Read the model definition and answer for the solid it produces. Units are mm, in the model's axes. A direction names the side the tool comes from. Coordinates: 2 decimals unless noted, no trailing zeros. Loops run counter-clockwise (first coordinate to the right, second up) from the corner with the lowest first, then second, coordinate; pieces in that order, holes last. Notation, with made-up numbers: M 72.25,13 L 110.25,13 A25 ccw 110.25,41 Z; hole C -23,54 d7. An arc over 180 degrees is marked long. One line per item, written item: value. Start each with the question number.
1. The part is cut by section D-D (x = -114.5). Write down the section's boundary in (y, z), then the cut area to 3 significant figures.
2. The part is cut by section B-B (x = -17). Write down the section's boundary in (y, z).
3. For faces 4 (the face through (-144, 110, -7)), 5 (the face through (-144, -110, -7)), 6 (the face through (131.93, -37.13, -4.93)), 7 (the face through (-161, -100, 0)), 8 (the face through (-144, -90, -7)), determine the directions among +Z, -Z, +X, -X, +Y, -Y from which every point of the face is accessible in a straight line to the end or side of a thin tool.
4. Determine the mould class of faces 1 (the face through (-2, -20, 0)), 2 (the face through (-177.26, 99.86, -14.67)), 3 (the face through (-146.445, -190.979, 7.395)) for opening direction X: +X half, -X half, draft (parallel to the pull), parting line (faces both ways), or undercut.
5. Flat-ended cylindrical pins translate along their axes: pin 1 (4 mm diameter, centred on x = 122.5, z = -12, fed in from -Y); pin 2 (4 mm diameter, centred on y = 21, z = -12.5, fed in from +X); pin 3 (10 mm diameter, centred on x = -158.5, y = -97, fed in from +Z); pin 4 (5 mm diameter, centred on y = 48, z = 2, fed in from -X). Find the tip coordinate at first contact, or state that the pin passes through.
6. The part is cut by section C-C (y = -66). Write down the section's boundary in (x, z), then the cut area to 3 significant figures.
7. Consider probe 1 along Z at (x, y) = (-167, -103); probe 2 along X at (y, z) = (-98, -12.5); probe 3 along Z at (x, y) = (-106, -58). Determine where each line is inside the solid, lowest interval first.
8. The part is cut by section A-A (y = 24). Write down the section's boundary in (x, z).
```python
from build123d import *

# Parameters (mm, degrees)
BOSS_EXTRUDE1_DEPTH      = 15
BOSS_EXTRUDE2_DEPTH      = 10
BOSS_EXTRUDE2_DEPTH_BACK = 10
SKETCH3_R                = 12.5
SKETCH3_R_2              = 10
BOSS_EXTRUDE3_DEPTH      = 10
BOSS_EXTRUDE3_DEPTH_BACK = 10
SKETCH4_R                = 12.5
SKETCH4_R_2              = 10
CUT_EXTRUDE1_DEPTH       = 46
SKETCH6_R                = 7.5
BOSS_EXTRUDE4_DEPTH      = 10
BOSS_EXTRUDE5_DEPTH      = 5


with BuildPart() as part:
    # Sketch1 → Boss-Extrude1 (new body)
    with BuildSketch(Plane.XY):
        Polygon((-155, 155), (-155, -200), (155, -200), (155, 81.722524266), (81.722524266, 155), align=None)
    extrude(amount=BOSS_EXTRUDE1_DEPTH)

    # Sketch3 → Boss-Extrude2 (add, two sides: drawn at the far end of the back side and taken through both)
    # profile 1 of 2: a face of its own
    with BuildSketch(Plane(origin=(0, 100, 0), x_dir=(1, 0, 0), z_dir=(0, 1, 0)).offset(-BOSS_EXTRUDE2_DEPTH_BACK)):
        with BuildLine():
            ThreePointArc((-155, 12.5), (-158.661165235, 3.661165235), (-167.5, 0))
            Line((-167.5, 0), (-107.5, 0))
            Line((-107.5, 0), (-162.508319468, 23.960066556))
            ThreePointArc((-162.508319468, 23.960066556), (-157.04423588, 19.350328216), (-155, 12.5))
        make_face()
    # profile 2 of 2: a face of its own
    with BuildSketch(Plane(origin=(0, 100, 0), x_dir=(1, 0, 0), z_dir=(0, 1, 0)).offset(-BOSS_EXTRUDE2_DEPTH_BACK)):
        with Locations((-167.5, 12.5)):
            Circle(SKETCH3_R)
        with Locations(Location((-167.5, 12.5, 0), (0, 0, 270))):
            Circle(SKETCH3_R_2, mode=Mode.SUBTRACT)
    extrude(amount=BOSS_EXTRUDE2_DEPTH + BOSS_EXTRUDE2_DEPTH_BACK)

    # Sketch4 → Boss-Extrude3 (add, two sides: drawn at the far end of the back side and taken through both)
    # profile 1 of 2: a face of its own
    with BuildSketch(Plane(origin=(0, -100, 0), x_dir=(1, 0, 0), z_dir=(0, 1, 0)).offset(-BOSS_EXTRUDE3_DEPTH_BACK)):
        with Locations((-167.5, 12.5)):
            Circle(SKETCH4_R)
        with Locations(Location((-167.5, 12.5, 0), (0, 0, 270))):
            Circle(SKETCH4_R_2, mode=Mode.SUBTRACT)
    # profile 2 of 2: a face of its own
    with BuildSketch(Plane(origin=(0, -100, 0), x_dir=(1, 0, 0), z_dir=(0, 1, 0)).offset(-BOSS_EXTRUDE3_DEPTH_BACK)):
        with BuildLine():
            Line((-107.5, 0), (-162.508319468, 23.960066556))
            ThreePointArc((-162.508319468, 23.960066556), (-157.04423588, 19.350328216), (-155, 12.5))
            ThreePointArc((-155, 12.5), (-158.661165235, 3.661165235), (-167.5, 0))
            Line((-167.5, 0), (-107.5, 0))
        make_face()
    extrude(amount=BOSS_EXTRUDE3_DEPTH + BOSS_EXTRUDE3_DEPTH_BACK)

    # Sketch5 → Cut-Extrude1 (cut)
    with BuildSketch(Plane(origin=(0, 0, 0), x_dir=(-1, 0, 0), z_dir=(0, 0, -1))):
        with BuildLine():
            ThreePointArc((-125, -200), (-146.213203436, -191.213203436), (-155, -170))
            Line((-155, -170), (-155, -200))
            Line((-155, -200), (-125, -200))
        make_face()
        with BuildLine():
            ThreePointArc((155, -170), (146.213203436, -191.213203436), (125, -200))
            Line((125, -200), (155, -200))
            Line((155, -200), (155, -170))
        make_face()
        with BuildLine():
            Line((155, 155), (125, 155))
            ThreePointArc((125, 155), (146.213203436, 146.213203436), (155, 125))
            Line((155, 125), (155, 155))
        make_face()
        with BuildLine():
            Line((-81.722524266, 155), (-90.50932083, 146.213203436))
            ThreePointArc((-90.50932083, 146.213203436), (-80.776620365, 152.716385975), (-69.296117394, 155))
            Line((-69.296117394, 155), (-81.722524266, 155))
        make_face()
        with BuildLine():
            ThreePointArc((-155, 69.296117394), (-152.716385975, 80.776620365), (-146.213203436, 90.50932083))
            Line((-146.213203436, 90.50932083), (-155, 81.722524266))
            Line((-155, 81.722524266), (-155, 69.296117394))
        make_face()
    extrude(amount=-CUT_EXTRUDE1_DEPTH, mode=Mode.SUBTRACT)

    # Sketch6 → Boss-Extrude4 (add)
    with BuildSketch(Plane(origin=(0, 0, 0), x_dir=(-1, 0, 0), z_dir=(0, 0, -1))):
        with Locations(Location((-125, 40, 0), (0, 0, 180))):
            Circle(SKETCH6_R)
        with Locations(Location((-125, -40, 0), (0, 0, 180))):
            Circle(SKETCH6_R)
    extrude(amount=BOSS_EXTRUDE4_DEPTH)

    # Sketch7 → Boss-Extrude5 (add)
    with BuildSketch(Plane(origin=(0, 0, -10), x_dir=(-1, 0, 0), z_dir=(0, 0, -1))):
        with BuildLine():
            Line((-130, 50), (-120, 50))
            ThreePointArc((-120, 50), (-116.464466094, 48.535533906), (-115, 45))
            Line((-115, 45), (-115, -45))
            ThreePointArc((-115, -45), (-116.464466094, -48.535533906), (-120, -50))
            Line((-120, -50), (-130, -50))
            ThreePointArc((-130, -50), (-133.535533906, -48.535533906), (-135, -45))
            Line((-135, -45), (-135, 45))
            ThreePointArc((-135, 45), (-133.535533906, 48.535533906), (-130, 50))
        make_face()
    extrude(amount=BOSS_EXTRUDE5_DEPTH)


solid = part.part
```
Answer block:
1. outline: M -200,0 L -110,0 L -110,-3.05 L -90,-3.05 L -90,0 L 90,0 L 90,-3.05 L 110,-3.05 L 110,0 L 155,0 L 155,15 L -200,15 Z
1. area: 5,450 mm2
2. outline: M -200,0 L 155,0 L 155,15 L -200,15 Z
3. face 4: -Z, +X, -X, +Y
3. face 5: -Z, +X, -X, -Y
3. face 6: none
3. face 7: +Z, -X, +Y, -Y
3. face 8: -Z, +X, -X
4. face 1: draft
4. face 2: undercut
4. face 3: -X half
5. pin 1: stops at y = -50
5. pin 2: stops at x = 135
5. pin 3: stops at z = 15
5. pin 4: stops at x = -155
6. outline: M -155,0 L 155,0 L 155,15 L -155,15 Z
6. area: 4,650 mm2
7. probe 1: z = -24.99 to -22.49, -2.51 to 0
7. probe 2: x = -180 to -177.5, -157.5 to -136.2
7. probe 3: z = 0 to 15
8. outline: M -155,0 L 155,0 L 155,15 L -155,15 Z; M 115,-15 L 135,-15 L 135,-10 L 115,-10 Z
